Geometry: final body of the model. Coordinates: model frame, mm. Face numbers are marked on the shaded views. A direction names the side the tool comes from. Give positions to 0.01 mm unless a question says otherwise; leave off trailing zeros. Order: outer loops, then holes, each group sorted by start corner. A loop starts at its lowest first (then second) coordinate and runs counter-clockwise, first axis right, second up. Notation, with made-up numbers: (21.25, 10) - (69.25, 10) arc R15 cw to (69.25, 32) - close; hole circle Ø8 at (10.5, 31.5). An arc over 180 degrees is marked (long way). Use one line per item in the form item = value.
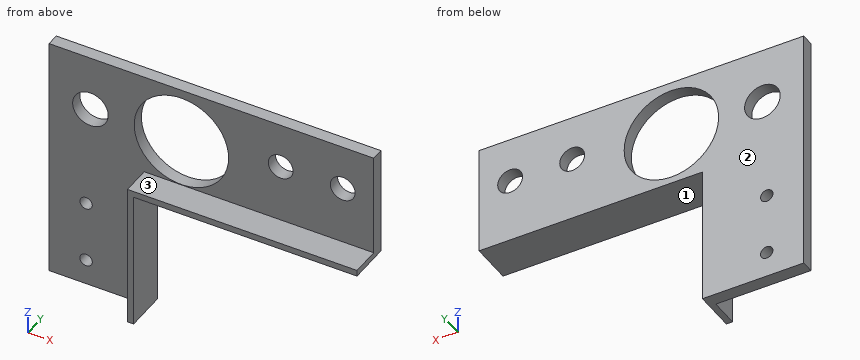
from build123d import *

# Parameters (mm, degrees)
SALIENTE_EXTRUIR1_DEPTH = 3
CROQUIS2_R              = 3
CROQUIS2_R_2            = 1.5
CORTAR_EXTRUIR2_DEPTH   = 4
SALIENTE_EXTRUIR2_DEPTH = 10
CROQUIS4_R              = 11.420621249
CORTAR_EXTRUIR3_DEPTH   = 11
CROQUIS5_W              = 78.5
CROQUIS5_H              = 3
SALIENTE_EXTRUIR3_DEPTH = 2
CROQUIS6_R              = 4.304654485
CORTAR_EXTRUIR4_DEPTH   = 11


with BuildPart() as part:
    # Croquis1 → Saliente-Extruir1 (new body)
    with BuildSketch(Plane(origin=(0, 0, 0), x_dir=(1, 0, 0), z_dir=(0, 1, 0))):
        Polygon((-16.25, 29), (-16.25, -6), (39.25, -6), (39.25, -29), (-39.25, -29), (-39.25, 29), align=None)
    extrude(amount=SALIENTE_EXTRUIR1_DEPTH)

    # Croquis2 → Cortar-Extruir2 (cut, through all)
    with BuildSketch(Plane(origin=(0, 3, 0), x_dir=(1, 0, 0), z_dir=(0, 1, 0))):
        with Locations((31.75, -20.05)):
            Circle(CROQUIS2_R)
        with Locations((16.75, -20.05)):
            Circle(CROQUIS2_R)
        with Locations((-30.3, 22.75)):
            Circle(CROQUIS2_R_2)
        with Locations((-30.3, 7.75)):
            Circle(CROQUIS2_R_2)
    extrude(amount=-CORTAR_EXTRUIR2_DEPTH, mode=Mode.SUBTRACT)

    # Croquis3 → Saliente-Extruir2 (add)
    with BuildSketch(Plane(origin=(0, 3, 0), x_dir=(1, 0, 0), z_dir=(0, 1, 0))):
        Polygon((-16.25, 29), (-16.25, -6), (39.25, -6), (39.25, -4.5), (-14.75, -4.5), (-14.75, 29), align=None)
    extrude(amount=-SALIENTE_EXTRUIR2_DEPTH)

    # Croquis4 → Cortar-Extruir3 (cut, through all)
    with BuildSketch(Plane(origin=(0, 3, 0), x_dir=(1, 0, 0), z_dir=(0, 1, 0))):
        with Locations((-7.25, -17.5)):
            Circle(CROQUIS4_R)
    extrude(amount=-CORTAR_EXTRUIR3_DEPTH, mode=Mode.SUBTRACT)

    # Croquis5 → Saliente-Extruir3 (add)
    with BuildSketch(Plane.XY.offset(29)):
        with Locations((0, 1.5)):
            Rectangle(CROQUIS5_W, CROQUIS5_H)
    extrude(amount=SALIENTE_EXTRUIR3_DEPTH)

    # Croquis6 → Cortar-Extruir4 (cut, through all)
    with BuildSketch(Plane(origin=(0, 3, 0), x_dir=(1, 0, 0), z_dir=(0, 1, 0))):
        with Locations((-29.25, -17.5)):
            Circle(CROQUIS6_R)
    extrude(amount=-CORTAR_EXTRUIR4_DEPTH, mode=Mode.SUBTRACT)


solid = part.part
(1) Cut plane D-D on y = -4. Output: boundary loops of the cut face in (x, z), plus the area to 4 significant figures.
Computed values:
outline = (-16.25, -29) - (-14.75, -29) - (-14.75, 4.5) - (39.25, 4.5) - (39.25, 6) - (-16.25, 6) - close
area = 133.5 mm²
(2) Cut plane C-C on z = 20.05. Output: boundary loops of the cut face in (x, y), plus the area to 3 significant figures.
Computed values:
outline = (-39.25, 0) - (-32.72, 0) - (-32.72, 3) - (-39.25, 3) - close; (-25.78, 0) - (-18.38, 0) - (-18.38, 3) - (-25.78, 3) - close; (3.88, 0) - (13.75, 0) - (13.75, 3) - (3.88, 3) - close; (19.75, 0) - (28.75, 0) - (28.75, 3) - (19.75, 3) - close; (34.75, 0) - (39.25, 0) - (39.25, 3) - (34.75, 3) - close
area = 112 mm²
(3) Cut plane B-B on x = 16.75. Output: boundary loops of the cut face in (y, z).
Computed values:
outline = (-7, 4.5) - (3, 4.5) - (3, 17.05) - (0, 17.05) - (0, 6) - (-7, 6) - close; (0, 23.05) - (3, 23.05) - (3, 31) - (0, 31) - close
(4) Contact query for flat-ended pins moving along their axis: pin 1 Ø7.5 at (x, z) = (-29.25, 17.5) entering from +Y; pin 2 Ø5 at (x, y) = (2.5, -0.5) entering from -Z; pin 3 Ø5 at (x, z) = (-30.3, -22.75) entering from -Y; pin 4 Ø4 at (y, z) = (0, -16) entering from +X. Output: stop coordinate, or through.
Computed values:
pin_1 = through
pin_2 = 4.5
pin_3 = 0
pin_4 = -14.75
(5) Ray query, line 1 along X through (y, z) = (1.05, -22.75); line 2 along Z through (x, y) = (-29.25, 1.45); line 3 along X through (y, z) = (1.6, 17.5). Return the intervals inside material, ascending.
Computed values:
line_1 = -39.25 to -31.8, -28.8 to -14.75
line_2 = -29 to -23.82, -21.68 to -8.82, -6.68 to 13.2, 21.8 to 31
line_3 = -39.25 to -33.55, -24.95 to -18.67, 4.17 to 15.17, 18.33 to 30.17, 33.33 to 39.25
(6) Reachability of the marked faces 1, 2 and 3 from +Z, -Z, +X, -X, +Y, -Y: full face, straight path, thin tool, end or side. Return the list, or none.
Computed values:
face_1 = -Z, +X, +Y, -Y
face_2 = +Z, -Z, +X, -X, +Y
face_3 = +Z, +X, -X, -Y
(7) Cut plane A-A on z = -22.75. Output: boundary loops of the cut face in (x, y), plus the area to 3 significant figures.
Computed values:
outline = (-39.25, 0) - (-31.8, 0) - (-31.8, 3) - (-39.25, 3) - close; (-28.8, 0) - (-16.25, 0) - (-16.25, -7) - (-14.75, -7) - (-14.75, 3) - (-28.8, 3) - close
area = 75.0 mm²
